Work out the finished part from the listing and answer in its coordinate system (mm). Give positions to 0.01 mm unless a question says otherwise; leave off trailing zeros. Loops run counter-clockwise (first coordinate to the right, second up) from the corner with the lowest first, then second, coordinate; pieces in that order, holes last. Notation, with made-up numbers: (-38, -22.5) - (-30, -22.5) arc R15 ccw to (-30, -14.5) - close; hole circle Ø9 at (70, -11.75). An arc over 180 degrees is marked (long way). One line per question, with ' | ' between items.
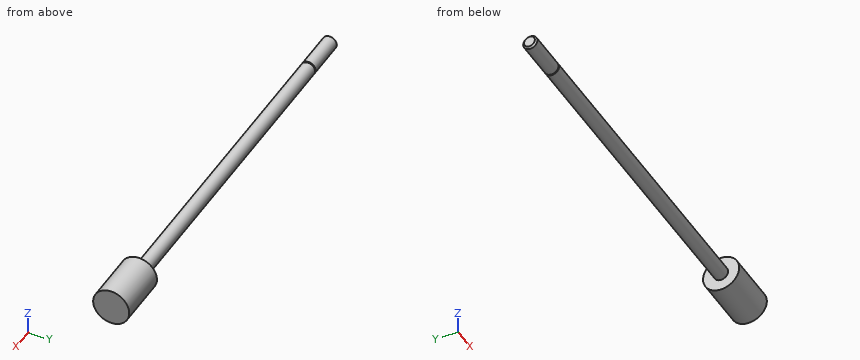
Autodesk Inventor part; units mm, degrees
ref_plane "rod_cp_XY" through (0, 0, 0) normal (1, 0, 0) x (0, 0, -1)
ref_plane "rod_cp_YZ" through (0, 0, 0) normal (0, 0, -1) x (0, 1, 0)
ref_plane "rod_cp_ZX" through (0, 0, 0) normal (0, 1, 0) x (1, 0, 0)
sketch "Sketch_1" plane through (0, 0, 0) normal (0, 0, 1) x (1, 0, 0)
  line L0 (84.0994, 0) -> (0, 0)
  line L1 (0, 0) -> (0, 1.5875)
  line L2 (0, 1.5875) -> (72.263, 1.5875)
  line L3 (72.263, 1.5875) -> (72.263, 4.0323)
  line L4 (72.263, 4.0323) -> (84.0994, 4.0323)
  line L5 (84.0994, 4.0323) -> (84.0994, 0)
  line L6 (84.0994, 0) -> (0, 0)
revolve "Revolution1" add sketch "Sketch_1" angle 360 about axis through (84.0994, 0, 0) along (1, 0, 0)
sketch "Sketch_2" plane through (0, 0, 0) normal (0, 0, 1) x (1, 0, 0)
  line L0 (0, 0) -> (-9.652, 0)
  line L1 (-9.652, 0) -> (-9.652, 1.209)
  line L2 (-9.652, 1.209) -> (-9.2735, 1.5875)
  line L3 (-9.2735, 1.5875) -> (0, 1.5875)
  line L4 (0, 1.5875) -> (0, 0)
  line L5 (0, 0) -> (-9.652, 0)
revolve "Revolution2" add sketch "Sketch_2" angle 360 about axis through (0, 0, 0) along (1, 0, 0)
sketch "Sketch_30" plane through (0, 0, 0) normal (0, 0, 1) x (1, 0, 0)
  line L0 (0, 0) -> (-0.254, 0)
  line L1 (-0.254, 1.8415) -> (-0.254, 1.3335)
  line L2 (-0.254, 1.3335) -> (0, 1.3335)
  line L3 (0, 1.3335) -> (0, 1.8415)
  line L4 (0, 1.8415) -> (-0.254, 1.8415)
revolve "Revolution3" cut sketch "Sketch_30" angle 360 about axis through (0, 0, 0) along (1, 0, 0)
ref_plane "rod_cp_XY" through (0, 0, 0) normal (1, 0, 0) x (0, 0, -1)
ref_plane "rod_cp_YZ" through (0, 0, 0) normal (0, 0, -1) x (0, 1, 0)
ref_plane "rod_cp_ZX" through (0, 0, 0) normal (0, 1, 0) x (1, 0, 0)
ref_plane "to_rod_clevis_XY" through (-9.652, 0, 0) normal (1, 0, 0) x (0, 0, -1)
ref_plane "to_rod_clevis_YZ" through (-9.652, 0, 0) normal (0, 0, -1) x (0, 1, 0)
ref_plane "to_rod_clevis_ZX" through (-9.652, 0, 0) normal (0, 1, 0) x (1, 0, 0)
ref_plane "rl2_XY" through (0, 0, 0) normal (1, 0, 0) x (0, 0, -1)
ref_plane "rl2_YZ" through (0, 0, 0) normal (0, 0, -1) x (0, 1, 0)
ref_plane "rl2_ZX" through (0, 0, 0) normal (0, 1, 0) x (1, 0, 0)
ref_plane "rl1_XY" through (-9.652, 0, 0) normal (1, 0, 0) x (0, 0, -1)
ref_plane "rl1_YZ" through (-9.652, 0, 0) normal (0, 0, -1) x (0, 1, 0)
ref_plane "rl1_ZX" through (-9.652, 0, 0) normal (0, 1, 0) x (1, 0, 0)
ref_plane "thd1_XY" through (-9.652, 1.5875, 0) normal (1, 0, 0) x (0, 0, -1)
ref_plane "thd1_YZ" through (-9.652, 1.5875, 0) normal (0, 0, -1) x (0, 1, 0)
ref_plane "thd1_ZX" through (-9.652, 1.5875, 0) normal (0, 1, 0) x (1, 0, 0)
ref_plane "thd2_XY" through (-9.652, -1.5875, 0) normal (1, 0, 0) x (0, 0, -1)
ref_plane "thd2_YZ" through (-9.652, -1.5875, 0) normal (0, 0, -1) x (0, 1, 0)
ref_plane "thd2_ZX" through (-9.652, -1.5875, 0) normal (0, 1, 0) x (1, 0, 0)
ref_plane "dia1_XY" through (0, 1.5875, 0) normal (1, 0, 0) x (0, 0, -1)
ref_plane "dia1_YZ" through (0, 1.5875, 0) normal (0, 0, -1) x (0, 1, 0)
ref_plane "dia1_ZX" through (0, 1.5875, 0) normal (0, 1, 0) x (1, 0, 0)
ref_plane "dia2_XY" through (0, -1.5875, 0) normal (1, 0, 0) x (0, 0, -1)
ref_plane "dia2_YZ" through (0, -1.5875, 0) normal (0, 0, -1) x (0, 1, 0)
ref_plane "dia2_ZX" through (0, -1.5875, 0) normal (0, 1, 0) x (1, 0, 0)
ref_plane "dia1r_XY" through (0, 0, 5.5626) normal (1, 0, 0) x (0, 0, -1)
ref_plane "dia1r_YZ" through (0, 0, 5.5626) normal (0, 0, -1) x (0, 1, 0)
ref_plane "dia1r_ZX" through (0, 0, 5.5626) normal (0, 1, 0) x (1, 0, 0)
ref_plane "dia2r_XY" through (0, 0, -5.5626) normal (1, 0, 0) x (0, 0, -1)
ref_plane "dia2r_YZ" through (0, 0, -5.5626) normal (0, 0, -1) x (0, 1, 0)
ref_plane "dia2r_ZX" through (0, 0, -5.5626) normal (0, 1, 0) x (1, 0, 0)
ref_plane "dia12_XY" through (0, 0, 7.6835) normal (1, 0, 0) x (0, 0, -1)
ref_plane "dia12_YZ" through (0, 0, 7.6835) normal (0, 0, -1) x (0, 1, 0)
ref_plane "dia12_ZX" through (0, 0, 7.6835) normal (0, 1, 0) x (1, 0, 0)
ref_plane "dia22_XY" through (0, 0, -7.6835) normal (1, 0, 0) x (0, 0, -1)
ref_plane "dia22_YZ" through (0, 0, -7.6835) normal (0, 0, -1) x (0, 1, 0)
ref_plane "dia22_ZX" through (0, 0, -7.6835) normal (0, 1, 0) x (1, 0, 0)
properties part number "0072-DXP0_rod"
1. Consider L1, parallel to X at y = 0.25, z = -2; L2, parallel to X at y = -1.25, z = -0.75; L3, parallel to Z at x = 41, y = -0.25. Determine where each line is inside the solid, lowest interval first.
Evaluation:
L1: 72.26 to 84.1 | L2: -9.4 to -0.25, 0 to 84.1 | L3: -1.57 to 1.57
2. Find section C-C on x = 60.5. Write down the section's boundary in (y, z) (1 decimal), then the cut area to 3 significant figures.
Evaluation:
outline: circle Ø3.2 at (0, 0) | area: 7.92 mm2
3. Find section A-A on z = 0. Write down the section's boundary in (x, y), then the cut area to 3 significant figures.
Evaluation:
outline: (-9.65, -1.21) - (-9.27, -1.59) - (-0.25, -1.59) - (-0.25, -1.33) - (0, -1.33) - (0, -1.59) - (72.26, -1.59) - (72.26, -4.03) - (84.1, -4.03) - (84.1, 4.03) - (72.26, 4.03) - (72.26, 1.59) - (0, 1.59) - (0, 1.33) - (-0.25, 1.33) - (-0.25, 1.59) - (-9.27, 1.59) - (-9.65, 1.21) - close | area: 355 mm2
4. Flat-ended cylindrical pins translate along their axes: pin 1 (2 mm diameter, centred on x = 39.5, z = 1, fed in from -Y); pin 2 (2 mm diameter, centred on x = 17, y = 2, fed in from +Z); pin 3 (4 mm diameter, centred on x = 71.5, z = 2, fed in from +Y). Find the tip coordinate at first contact, or state that the pin passes through.
Evaluation:
pin 1: y = -1.59 | pin 2: z = 1.23 | pin 3: y = 4.03
